Work out the finished part from the listing and answer in its coordinate system (mm). A direction names the side the tool comes from. Give positions to 0.01 mm unless a question says otherwise; leave off trailing zeros. Loops run counter-clockwise (first coordinate to the right, second up) from the corner with the lowest first, then second, coordinate; pieces in that order, holes last. Notation, with made-up numbers: (39.25, 24) - (56.25, 24) arc R15 ccw to (56.25, 35) - close; hole circle Ø10 at (22.25, -6.5). An arc over 180 degrees is marked (long way). One line per question, with ' | ' between items. Start each with the question number.
1. Which of the six approach directions +Z, -Z, +X, -X, +Y, -Y give full straight-line access (tool end or side, diameter ignored) to faces 1 (the face through (2.704, 4.634, 0.74)), 2 (the face through (6, 0, 0))?
2. For a pull along Y with two mould halves and no side action, classify faces 3 (the face through (-2.74, -4.68, 0.74)), 4 (the face through (-29.97, 1.32, 0.74)), 5 (the face through (6, 0, 1.5)) as released by +Y, released by -Y, zero draft, split by the parting line, or undercut.
3. Section B-B (z = 0.85) is taken. Determine the outline of the cut face in (x, y).
4. Section D-D (x = 21.5) is taken. Determine the outline of the cut face in (y, z).
5. Section A-A (x = 15) is taken. Determine the outline of the cut face in (y, z), plus the area to 3 significant figures.
6. Find the intervals of material crossed by line 1 (Y direction, x = -7.5, z = 0.5); line 2 (Y direction, x = 5.5, z = 0.15); line 3 (X direction, y = 7.5, z = 1.3), in increasing order.
7. Section C-C (y = 22.5) is taken. Determine the outline of the cut face in (x, z), plus the area to 3 significant figures.
from build123d import *

# Parameters (mm, degrees)
SKETCH1_R           = 30
SKETCH1_R_2         = 2
BOSS_EXTRUDE1_DEPTH = 1.5
CUT_EXTRUDE1_DEPTH  = 10
FILLET1_R           = 2


with BuildPart() as part:
    # Sketch1 → Boss-Extrude1 (new body)
    with BuildSketch(Plane.XY):
        Circle(SKETCH1_R)
        with Locations((15, 0)):
            Circle(SKETCH1_R_2, mode=Mode.SUBTRACT)
        with Locations((-15, 0)):
            Circle(SKETCH1_R_2, mode=Mode.SUBTRACT)
    extrude(amount=BOSS_EXTRUDE1_DEPTH)

    # Sketch2 → Cut-Extrude1 (cut)
    with BuildSketch(Plane(origin=(0, 0, 0), x_dir=(-1, 0, 0), z_dir=(0, 0, -1))):
        Polygon((-12.124355653, -7), (-3.464101615, 2), (0, 14), (3.464101615, 2), (12.124355653, -7), (0, -4), align=None)
    extrude(amount=-CUT_EXTRUDE1_DEPTH, mode=Mode.SUBTRACT)

    # Fillet1
    fillet1_edges = [part.edges().sort_by_distance(p)[0] for p in [
        (-12.124355653, -7, 0.75),
        (12.124355653, -7, 0.75),
        (0, 14, 0.75),
    ]]
    fillet(fillet1_edges, radius=FILLET1_R)


solid = part.part
Conclusion:
1) face 1: +Z, -Z | face 2: -Z, +X, -X, +Y, -Y
2) face 3: undercut | face 4: split by the parting line | face 5: zero draft
3) outline: circle Ø60 at (0, 0); hole circle Ø4 at (-15, 0); hole (-7.32, -2.01) arc R2 ccw to (-5.4, -5.34) - (0, -4) - (5.4, -5.34) arc R2 ccw to (7.32, -2.01) - (3.46, 2) - (1.92, 7.34) arc R2 ccw to (-1.92, 7.34) - (-3.46, 2) - close; hole circle Ø4 at (15, 0)
4) outline: (-20.92, 0) - (20.92, 0) - (20.92, 1.5) - (-20.92, 1.5) - close
5) outline: (-25.98, 0) - (-2, 0) - (-2, 1.5) - (-25.98, 1.5) - close; (2, 0) - (25.98, 0) - (25.98, 1.5) - (2, 1.5) - close | area: 71.9 mm²
6) line 1: -29.05 to -4.57, -2.22 to 29.05 | line 2: -29.49 to -5.36, -0.12 to 29.49 | line 3: -29.05 to -1.87, 1.87 to 29.05
7) outline: (-19.84, 0) - (19.84, 0) - (19.84, 1.5) - (-19.84, 1.5) - close | area: 59.5 mm²
